Source: CAD feature listing. Evaluate the final solid. Frame: model axes, mm. A direction names the side the tool comes from. Coordinates: 2 decimals unless noted, no trailing zeros. Write each loop counter-clockwise with the first axis right and the second up, starting at its lowest first coordinate (ties: lowest second). Pieces come first, ordered by that corner, then holes. Notation, with made-up numbers: (26, 77) -> (48, 77) arc R15 cw to (48, 88) -> close; hole circle Ø5 at (-21.75, 21.25). An arc over 180 degrees is marked (long way). Write item = value, one per line.
from build123d import *

# Parameters (mm, degrees)
ESQUISSE1_R             = 2.5
BOSS_EXTRU_1_DEPTH      = 3
ESQUISSE2_W             = 20
ESQUISSE2_H             = 10
ENL_V_MAT_EXTRU_1_DEPTH = 174.720827721
SKETCH1_W               = 235.08624341
SKETCH1_H               = 3
BOSS_EXTRUDE1_DEPTH     = 20
CUT_EXTRUDE1_DEPTH      = 10
SKETCH3_W               = 20
SKETCH3_H               = 2.74057888
CUT_EXTRUDE2_DEPTH      = 10


with BuildPart() as part:
    # Esquisse1 → Boss.-Extru.1 (new body)
    with BuildSketch(Plane(origin=(0, 0, 0), x_dir=(1, 0, 0), z_dir=(0, 1, 0))):
        Polygon((-170.028456395, 18.77), (-170.028456395, -23), (-170.028456395, -35.5), (110.271543605, -35.5), (110.271543605, -10.5), (65.057787015, -10.5), (65.057787015, 28.77), (-170.028456395, 28.77), align=None)
        with Locations(Location((100.471543605, -23, 0), (0, 0, 270))):
            Circle(ESQUISSE1_R, mode=Mode.SUBTRACT)
        with Locations(Location((-160.228456395, -19.4325, 0), (0, 0, 270))):
            Circle(ESQUISSE1_R, mode=Mode.SUBTRACT)
        with Locations(Location((-160.228456395, 12.7025, 0), (0, 0, 270))):
            Circle(ESQUISSE1_R, mode=Mode.SUBTRACT)
        with Locations(Location((44.807787015, 10.747499922, 0), (0, 0, 270))):
            Circle(ESQUISSE1_R, mode=Mode.SUBTRACT)
    extrude(amount=BOSS_EXTRU_1_DEPTH)

    # Esquisse2 → Enlèv. mat.-Extru.1 (cut, through all)
    with BuildSketch(Plane(origin=(0, 3, 0), x_dir=(1, 0, 0), z_dir=(0, 1, 0))):
        with BuildLine():
            Line((-113.756895542, 11.635), (-113.756895542, -18.365))
            ThreePointArc((-113.756895542, -18.365), (-111.256895542, -20.865), (-108.756895542, -18.365))
            Line((-108.756895542, -18.365), (-108.756895542, 11.635))
            ThreePointArc((-108.756895542, 11.635), (-111.256895542, 14.135), (-113.756895542, 11.635))
        make_face()
        with BuildLine():
            Line((-54.98533469, 11.635), (-54.98533469, -18.365))
            ThreePointArc((-54.98533469, -18.365), (-52.48533469, -20.865), (-49.98533469, -18.365))
            Line((-49.98533469, -18.365), (-49.98533469, 11.635))
            ThreePointArc((-49.98533469, 11.635), (-52.48533469, 14.135), (-54.98533469, 11.635))
        make_face()
        with BuildLine():
            Line((3.786226163, 11.635), (3.786226163, -18.365))
            ThreePointArc((3.786226163, -18.365), (6.286226163, -20.865), (8.786226163, -18.365))
            Line((8.786226163, -18.365), (8.786226163, 11.635))
            ThreePointArc((8.786226163, 11.635), (6.286226163, 14.135), (3.786226163, 11.635))
        make_face()
        with Locations((75.271543605, -23)):
            Rectangle(ESQUISSE2_W, ESQUISSE2_H)
    extrude(amount=-ENL_V_MAT_EXTRU_1_DEPTH, mode=Mode.SUBTRACT)

    # Sketch1 → Boss-Extrude1 (add)
    with BuildSketch(Plane(origin=(0, 0, -28.77), x_dir=(-1, 0, 0), z_dir=(0, 0, -1))):
        with Locations((52.48533469, 1.5)):
            Rectangle(SKETCH1_W, SKETCH1_H)
    extrude(amount=BOSS_EXTRUDE1_DEPTH)

    # Sketch2 → Cut-Extrude1 (cut)
    with BuildSketch(Plane(origin=(0, 0, 0), x_dir=(-1, 0, 0), z_dir=(0, -1, 0))):
        with BuildLine():
            Line((99.256895542, -18.365), (99.256895542, 31.635))
            ThreePointArc((99.256895542, 31.635), (111.256895542, 43.635), (123.256895542, 31.635))
            Line((123.256895542, 31.635), (123.256895542, -18.365))
            ThreePointArc((123.256895542, -18.365), (111.256895542, -30.365), (99.256895542, -18.365))
        make_face()
        with BuildLine():
            Line((39.256895542, -18.365), (39.256895542, 31.635))
            ThreePointArc((39.256895542, 31.635), (51.256895542, 43.635), (63.256895542, 31.635))
            Line((63.256895542, 31.635), (63.256895542, -18.365))
            ThreePointArc((63.256895542, -18.365), (51.256895542, -30.365), (39.256895542, -18.365))
        make_face()
        with BuildLine():
            Line((-20.743104458, -18.365), (-20.743104458, 31.635))
            ThreePointArc((-20.743104458, 31.635), (-8.743104458, 43.635), (3.256895542, 31.635))
            Line((3.256895542, 31.635), (3.256895542, -18.365))
            ThreePointArc((3.256895542, -18.365), (-8.743104458, -30.365), (-20.743104458, -18.365))
        make_face()
    extrude(amount=-CUT_EXTRUDE1_DEPTH, mode=Mode.SUBTRACT)

    # Sketch3 → Cut-Extrude2 (cut)
    with BuildSketch(Plane(origin=(0, 3, 0), x_dir=(1, 0, 0), z_dir=(0, 1, 0))):
        Polygon((85.271543605, -28), (85.271543605, -30.74057888), (91.436540381, -30.74057888), (91.436540381, -15.25942112), (85.271543605, -15.25942112), (85.271543605, -18), align=None)
        with Locations((75.271543605, -16.62971056)):
            Rectangle(SKETCH3_W, SKETCH3_H)
        with Locations((75.271543605, -29.37028944)):
            Rectangle(SKETCH3_W, SKETCH3_H)
    extrude(amount=-CUT_EXTRUDE2_DEPTH, mode=Mode.SUBTRACT)


solid = part.part
1) Cut plane D-D, the plane x = -115. Output: boundary loops of the cut face in (y, z).
Answer block:
outline = (0, -48.77) -> (3, -48.77) -> (3, -43.04) -> (0, -43.04) -> close; (0, 29.77) -> (3, 29.77) -> (3, 35.5) -> (0, 35.5) -> close
2) First-contact query: pin 1 Ø1 at (y, z) = (1, -34) entering from +X; pin 2 Ø1.5 at (x, y) = (89, 2) entering from -Z. Flat tips, straight axial feed; report the tip coordinate or a pass-through.
Answer block:
pin_1 = 65.06
pin_2 = 10.5
3) Pull-direction query (X, two-part tool) for faces 1 (the flat face through (-28, 0, -6)), 2 (the cylindrical face through (-51.521, 1.479, 30.362)); classes: +X half, -X half, draft (parallel to the pull), parting line (faces both ways), or undercut.
Answer block:
face_1 = draft
face_2 = undercut
4) Cut plane C-C, the plane y = 0.6. Give the number of separate pieces and of enclosed holes in the cut face, and give its area (3 significant figures).
Answer block:
separate_pieces = 1
enclosed_holes = 8
area = 15,500 mm2
5) Cut plane B-B, the plane z = -5.5. Output: boundary loops of the cut face in (x, y).
Answer block:
outline = (-170.03, 0) -> (-123.26, 0) -> (-123.26, 3) -> (-170.03, 3) -> close; (-99.26, 0) -> (-63.26, 0) -> (-63.26, 3) -> (-99.26, 3) -> close; (-39.26, 0) -> (-3.26, 0) -> (-3.26, 3) -> (-39.26, 3) -> close; (20.74, 0) -> (65.06, 0) -> (65.06, 3) -> (20.74, 3) -> close
6) Cut plane A-A, the plane x = 7. Output: boundary loops of the cut face in (y, z), and give its area (3 significant figures).
Answer block:
outline = (0, -48.77) -> (3, -48.77) -> (3, -43.51) -> (0, -43.51) -> close; (0, 30.24) -> (3, 30.24) -> (3, 35.5) -> (0, 35.5) -> close
area = 31.6 mm2
7) Material intervals for probe 1 along X at (y, z) = (2.1, 5.5); probe 2 along X at (y, z) = (1.7, -40.5); probe 3 along Z at (x, y) = (83, 0.65), sorted ascending. Write a range as [from, to].
Answer block:
probe_1 = [-170.03, -123.26], [-99.26, -63.26], [-39.26, -3.26], [20.74, 65.06]
probe_2 = [-170.03, -119.34], [-103.17, -59.34], [-43.17, 0.66], [16.83, 65.06]
probe_3 = [10.5, 15.26], [30.74, 35.5]
8) Reachability of faces 3 (the cylindrical face through (-110.993, 1.479, -43.632)), 4 (the flat face through (-28, 3, -6)) from +Z, -Z, +X, -X, +Y, -Y: full face, straight path, thin tool, end or side. Return the list, or none.
Answer block:
face_3 = +Y, -Y
face_4 = +Z, -Z, +X, -X, +Y
